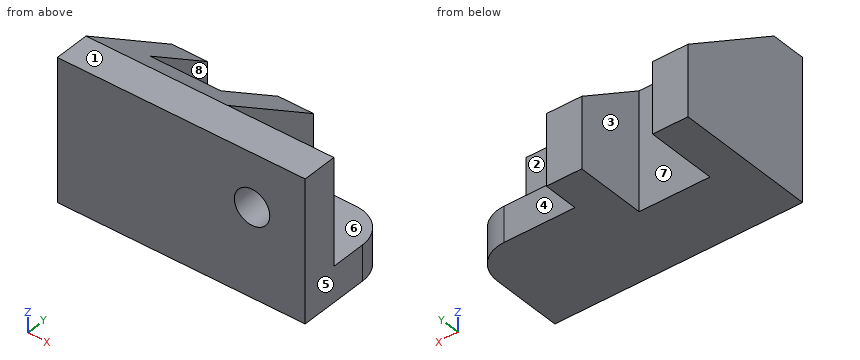
Autodesk Inventor part; units mm, degrees
ref_plane "YZ Plane" through (0, 0, 0) normal (1, 0, 0) x (0, 1, 0)
ref_plane "XZ Plane" through (0, 0, 0) normal (0, 1, 0) x (-1, 0, 0)
ref_plane "XY Plane" through (0, 0, 0) normal (0, 0, 1) x (1, 0, 0)
sketch "草圖1" plane through (0, 0, 0) normal (0, 1, 0) x (-1, 0, 0)
  line L0 (0, 0) -> (-70, 0)
  line L1 (-70, 0) -> (-70, -40)
  line L2 (-70, -40) -> (0, -40)
  line L3 (0, -40) -> (0, 0)
  dimension "d0" = 40
  dimension "d1" = 70
extrude "擠出1" add sketch "草圖1" along normal blind 10
sketch "草圖2" plane through (0, 0, 0) normal (0, 0, 1) x (1, 0, 0)
  line L0 (0, 0) -> (0, 10)
  line L1 (0, 10) -> (10, 10)
  line L2 (10, 10) -> (10, 40)
  line L3 (10, 40) -> (0, 40)
  line L4 (0, 40) -> (0, 10)
  line L5 (10, 10) -> (30, 10)
  line L6 (30, 10) -> (30, 20)
  line L7 (30, 20) -> (10, 20)
  line L8 (10, 20) -> (10, 10)
  line L9 (30, 10) -> (40, 10)
  line L10 (40, 10) -> (40, 40)
  line L11 (40, 40) -> (30, 40)
  line L12 (30, 40) -> (30, 10)
  dimension "d4" = 20
  dimension "d5" = 10
  dimension "d6" = 10
  dimension "d7" = 10
  dimension "d8" = 30
extrude "擠出2" add sketch "草圖2" against normal blind 40
sketch "草圖3" plane through (70, 0, -40) normal (0, 0, -1) x (-1, 0, 0)
  line L0 (30, 10) -> (30, 40)
  line L1 (30, 10) -> (0, 10)
  line L2 (0, 10) -> (0, 30)
  line L3 (0, 30) -> (30, 30)
  line L4 (30, 30) -> (30, 10)
  point P0 (70, 0)
  dimension "d11" = 20
  dimension "d12" = 30
extrude "擠出3" add sketch "草圖3" against normal blind 10
fillet "圓角1" radius 10 1 edges at (70, 30, -35)
sketch "草圖4" plane through (40, 10, 0) normal (1, 0, 0) x (0, 0, -1)
  line L0 (0, 0) -> (0, 30)
  line L1 (0, 0) -> (20, 30)
  line L2 (20, 30) -> (0, 30)
  point P0 (0, -10)
  dimension "d16" = 20
  dimension "d17" = 30
extrude "擠出4" cut sketch "草圖4" against normal through all
sketch "草圖5" plane through (0, 10, 0) normal (0, 1, 0) x (1, 0, 0)
  circle A0 centre (55, 15) radius 5
  line L0 (70, 0) -> (70, 30)
  line L1 (40, 0) -> (70, 0)
  point P0 (0, 0)
  dimension "d20" = 15
  dimension "d21" = 15
  dimension "d22" = 10
extrude "擠出5" cut sketch "草圖5" against normal blind 10
properties part number "31"
Part model, mm, in its own coordinate system. Face numbers are marked on the shaded views. A direction names the side the tool comes from. Coordinates: 2 decimals unless noted, no trailing zeros. Loops run counter-clockwise (first coordinate to the right, second up) from the corner with the lowest first, then second, coordinate; pieces in that order, holes last. Notation, with made-up numbers: (1.5, 26.25) - (51.5, 26.25) arc R25 ccw to (51.5, 43.25) - close; hole circle Ø1 at (57.25, 14.5). An arc over 180 degrees is marked (long way). Write item = value, one per line. Start each with the question number.
Item 1: Wall check: L1, parallel to Z at x = 55, y = 7; L2, parallel to X at y = 3, z = -15; L3, parallel to X at y = 28.5, z = -12.5. Give the ranges that are in metal, low to high. Write a range as from..to.
Item 2: Mould opens along X. For the marked faces 5, 6, 7 and 8 say: released by +X, released by -X, zero draft, split by the parting line, or undercut.
Item 3: Cut at C-C, the plane y = 23.5. Give the cut face in (x, z), and give its area (3 significant figures).
Item 4: Flat gauge pins, fed straight in: pin 1 Ø8 at (x, z) = (47.5, -33.5) entering from +Y; pin 2 Ø4 at (y, z) = (26, -23) entering from +X; pin 3 Ø10 at (x, z) = (54.5, -13) entering from +Y. Where does each tip first touch, or does it go through?
Item 5: Cut at A-A, the plane z = -15. Give the cut face in (x, y).
Item 6: 3-axis set-ups, long thin cutter, end or side, ignore diameter. For the marked faces 1, 2, 3 and 4: which of +Z, -Z, +X, -X, +Y, -Y reach the whole face in a straight line?
Item 7: Cut at B-B, the plane x = 55. Give the cut face in (y, z).
Item 8: Cut at D-D, the plane y = 3. Give the cut face in (x, z), and give its area (3 significant figures).
The answers:
q1.L1 = -40..-20, -10..0
q1.L2 = 0..50, 60..70
q1.L3 = 0..10, 30..40
q2.face_5 = released by +X
q2.face_6 = zero draft
q2.face_7 = undercut
q2.face_8 = undercut
q3.outline = (0, -40) - (10, -40) - (10, -9) - (0, -9) - close; (30, -40) - (69.37, -40) - (69.37, -30) - (40, -30) - (40, -9) - (30, -9) - close
q3.area = 914 mm2
q4.pin_1 = 30
q4.pin_2 = 40
q4.pin_3 = 10
q5.outline = (0, 0) - (50, 0) - (50, 10) - (40, 10) - (40, 32.5) - (30, 32.5) - (30, 20) - (10, 20) - (10, 32.5) - (0, 32.5) - close; (60, 0) - (70, 0) - (70, 10) - (60, 10) - close
q6.face_1 = +Z, +X, -X, +Y, -Y
q6.face_2 = +Z, +X, +Y
q6.face_3 = +Z, -Z, +Y
q6.face_4 = +Z, -Z, +X, +Y
q7.outline = (0, -40) - (30, -40) - (30, -30) - (10, -30) - (10, -20) - (0, -20) - close; (0, -10) - (10, -10) - (10, 0) - (0, 0) - close
q8.outline = (0, -40) - (70, -40) - (70, 0) - (0, 0) - close; hole circle Ø10 at (55, -15)
q8.area = 2,720 mm2
